For this review, use the dimensioned drawing (mm, ordinates from the lowest corner) and the shaded views. A direction names the side the tool comes from. Coordinates: 2 decimals unless noted, no trailing zeros. Loops run counter-clockwise (first coordinate to the right, second up) from the corner with the lowest first, then second, coordinate; pieces in that order, holes last. Notation, with made-up numbers: (11, 87.5) - (41, 87.5) arc R18 ccw to (41, 97.5) - close; hole circle Ø7 at (24.5, 59.5). An arc over 180 degrees is marked (long way). Use a Markdown table: item, result. Add a question column.
1) The part is to be moulded in two halves that separate along Z. For the marked faces 6, 7 and 8, say which applies: pulls with the +Z half, pulls with the -Z half, needs draft (parallel to the pull), parting line crosses it, or undercut.
2) Add section A-A, the plane y = 4.25. Give the boundary of the cut face in (x, z).
3) Add section C-C, the plane x = 15. Give the boundary of the cut face in (y, z), and give its area (3 significant figures).
4) Clearance check with flat-ended pins moving along their axes: pin 1 (2.5 mm diameter, centred on x = 27.5, z = 2.5, fed in from +Y); pin 2 (1.9 mm diameter, centred on x = 26, z = 4, fed in from +Y); pin 3 (3 mm diameter, centred on x = 9.5, y = 5, fed in from +Z); pin 4 (10 mm diameter, centred on x = 9, y = 18.5, fed in from -Z). State where each tip first meets the part, or that it passes through.
5) To check wall thickness, follow L1, parallel to Z at x = 26, y = 3.55; L2, parallel to X at y = 9.5, z = 1.75; L3, parallel to Y at x = 27, z = 5.75. State the ranges of each line that lie inside material, in increasing order. Write a range as [from, to].
6) Add section B-B, the plane x = 26. Give the boundary of the cut face in (y, z), and give its area (3 significant figures).
7) Add section D-D, the plane z = 1. Give the boundary of the cut face in (x, y) (3 decimals), and give its area (3 significant figures).
8) For the marked faces 1, 2, 3, 4 and 5, list the 3-axis set-ups (+Z, -Z, +X, -X, +Y, -Y) from which the entire face can be reached by the end or side of a thin tool; tool diameter is ignored.
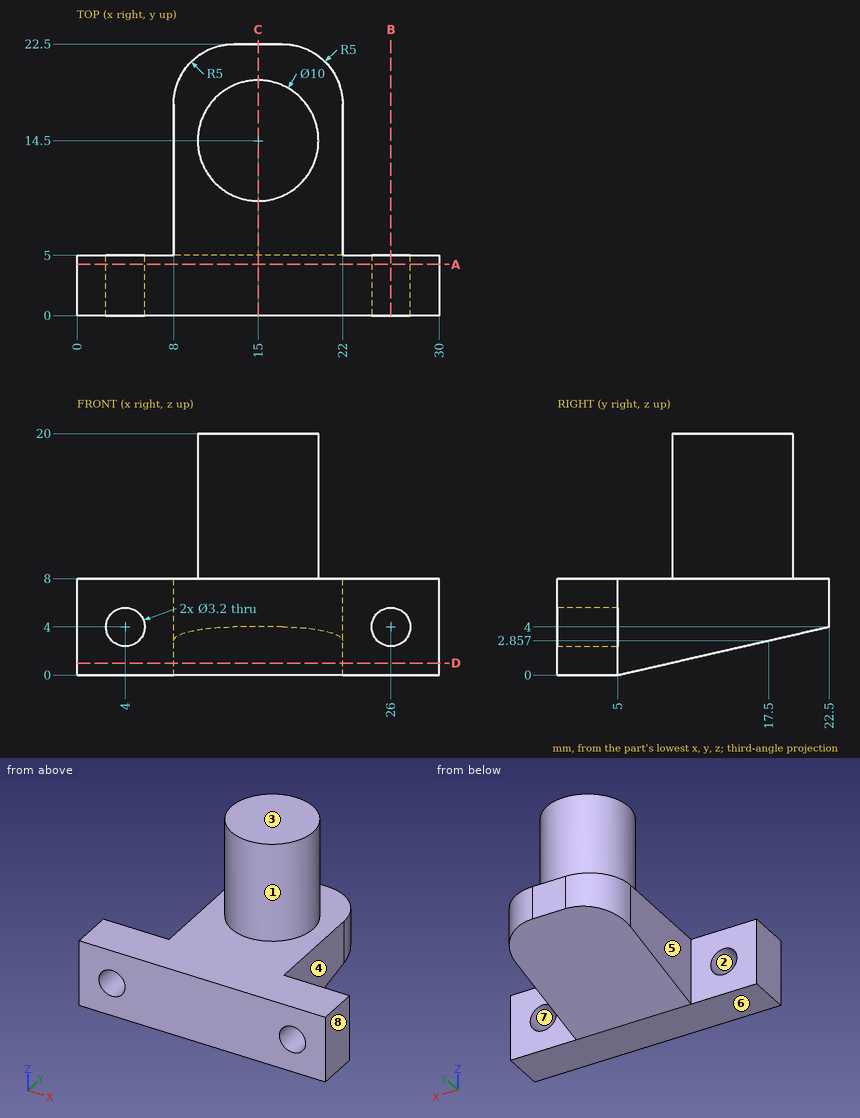
From the geometry:
| question | item | result |
|---|---|---|
| 1 | face 6 | pulls with the -Z half |
| 1 | face 7 | undercut |
| 1 | face 8 | needs draft |
| 2 | outline | (0, 0) - (30, 0) - (30, 8) - (0, 8) - close; hole circle Ø3.2 at (4, 4); hole circle Ø3.2 at (26, 4) |
| 3 | outline | (0, 0) - (5, 0) - (22.5, 4) - (22.5, 8) - (19.5, 8) - (19.5, 20) - (9.5, 20) - (9.5, 8) - (0, 8) - close |
| 3 | area | 265 mm^2 |
| 4 | pin 1 | stops at y = 5 |
| 4 | pin 2 | passes through |
| 4 | pin 3 | stops at z = 8 |
| 4 | pin 4 | stops at z = 1.94 |
| 5 | L1 | z = [0, 2.4], [5.6, 8] |
| 5 | L2 | x = [8, 22] |
| 5 | L3 | y = [0, 5] |
| 6 | outline | (0, 0) - (5, 0) - (5, 2.4) - (0, 2.4) - close; (0, 5.6) - (5, 5.6) - (5, 8) - (0, 8) - close |
| 6 | area | 24.0 mm^2 |
| 7 | outline | (0, 0) - (30, 0) - (30, 5) - (22, 5) - (22, 9.375) - (8, 9.375) - (8, 5) - (0, 5) - close |
| 7 | area | 211 mm^2 |
| 8 | face 1 | +Z |
| 8 | face 2 | +Y, -Y |
| 8 | face 3 | +Z, +X, -X, +Y, -Y |
| 8 | face 4 | +Z, -Z, +X, +Y |
| 8 | face 5 | +Z, -Z, -X, +Y |
